from build123d import *

# Parameters (mm, degrees)
SKETCH2_R           = 4.0005
CUT_EXTRUDE1_DEPTH  = 35.169146436
SKETCH3_R           = 6.35
SKETCH3_R_2         = 4.0005
BOSS_EXTRUDE1_DEPTH = 0.68072


with BuildPart() as part:
    # Sketch1 → Revolve1 (revolve)
    with BuildSketch(Plane.XY, mode=Mode.PRIVATE) as revolve1_sk:
        Polygon((0, 0), (0, 6.35), (5.1054, 6.35), (5.1054, 17.526), (8.2804, 17.526), (8.2804, 12.6746), (23.5204, 12.6746), (23.5204, 0), align=None)
    revolve(revolve1_sk.sketch.rotate(Axis((23.5204, 0, 0), (-1, 0, 0)), 90), axis=Axis((23.5204, 0, 0), (-1, 0, 0)))

    # Sketch2 → Cut-Extrude1 (cut, through all)
    with BuildSketch(Plane.ZY):
        Circle(SKETCH2_R)
    extrude(amount=-CUT_EXTRUDE1_DEPTH, mode=Mode.SUBTRACT)

    # Sketch3 → Boss-Extrude1 (add)
    with BuildSketch(Plane.ZY):
        with Locations(Location((0, 0, 0), (0, 0, 180))):
            Circle(SKETCH3_R)
        Circle(SKETCH3_R_2, mode=Mode.SUBTRACT)
    extrude(amount=BOSS_EXTRUDE1_DEPTH)


solid = part.part
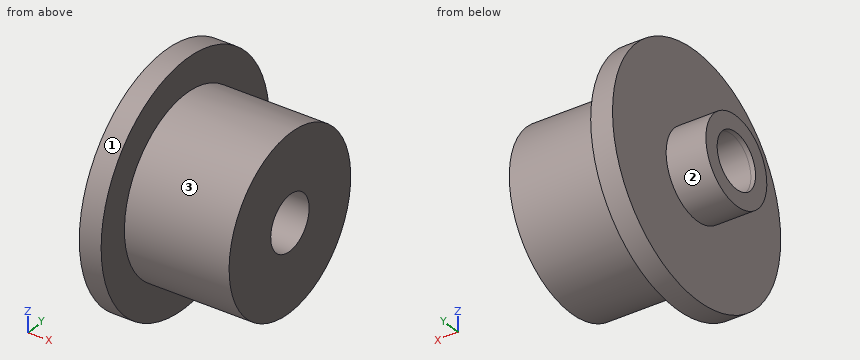
Source: CAD feature listing. Evaluate the final solid. Frame: model axes, mm. Face numbers are marked on the shaded views. A direction names the side the tool comes from. Coordinates: 2 decimals unless noted, no trailing zeros. Write each loop counter-clockwise with the first axis right and the second up, starting at its lowest first coordinate (ties: lowest second). Pieces come first, ordered by that corner, then holes. Notation, with made-up numbers: M 87,-9.5 L 102,-9.5 A22 ccw 102,17.5 Z; hole C -28.75,56.5 d4. An arc over 180 degrees is marked long. Use a Markdown table: item, result.
1) Reachability of the marked faces 1, 2 and 3 from +Z, -Z, +X, -X, +Y, -Y: full face, straight path, thin tool, end or side. Return the list, or none.
Conclusion:
| item | result |
|---|---|
| face 1 | +X, -X |
| face 2 | -X |
| face 3 | +X |
2) Ray query, L1, parallel to Y at x = 16, z = 0; L2, parallel to X at y = -2, z = -7; L3, parallel to X at y = -4, z = -12.5. Return the intervals inside material, ascending.
Conclusion:
| item | result |
|---|---|
| L1 | y = -12.67 to -4, 4 to 12.67 |
| L2 | x = 5.11 to 23.52 |
| L3 | x = 5.11 to 8.28 |
3) Section C-C, the plane x = 12.75. Output: boundary loops of the cut face in (y, z), then the cut area to 3 significant figures.
Conclusion:
| item | result |
|---|---|
| outline | C 0,0 d25.35; hole C 0,0 d8 |
| area | 454 mm^2 |
4) Section D-D, the plane z = -9.5. Output: boundary loops of the cut face in (x, y).
Conclusion:
| item | result |
|---|---|
| outline | M 5.11,-14.73 L 8.28,-14.73 L 8.28,-8.39 L 23.52,-8.39 L 23.52,8.39 L 8.28,8.39 L 8.28,14.73 L 5.11,14.73 Z |
5) First-contact query: pin 1 Ø5 at (y, z) = (13.5, 9.5) entering from -X; pin 2 Ø3 at (x, y) = (11, 2) entering from -Z; pin 3 Ø6 at (x, y) = (17.5, 10) entering from +Z. Flat tips, straight axial feed; report the tip coordinate or a pass-through.
Conclusion:
| item | result |
|---|---|
| pin 1 | stops at x = 5.11 |
| pin 2 | stops at z = -12.66 |
| pin 3 | stops at z = 10.57 |
6) Section A-A, the plane y = 0. Output: boundary loops of the cut face in (x, z).
Conclusion:
| item | result |
|---|---|
| outline | M -0.68,-6.35 L 5.11,-6.35 L 5.11,-17.53 L 8.28,-17.53 L 8.28,-12.67 L 23.52,-12.67 L 23.52,-4 L -0.68,-4 Z; M -0.68,4 L 23.52,4 L 23.52,12.67 L 8.28,12.67 L 8.28,17.53 L 5.11,17.53 L 5.11,6.35 L -0.68,6.35 Z |
